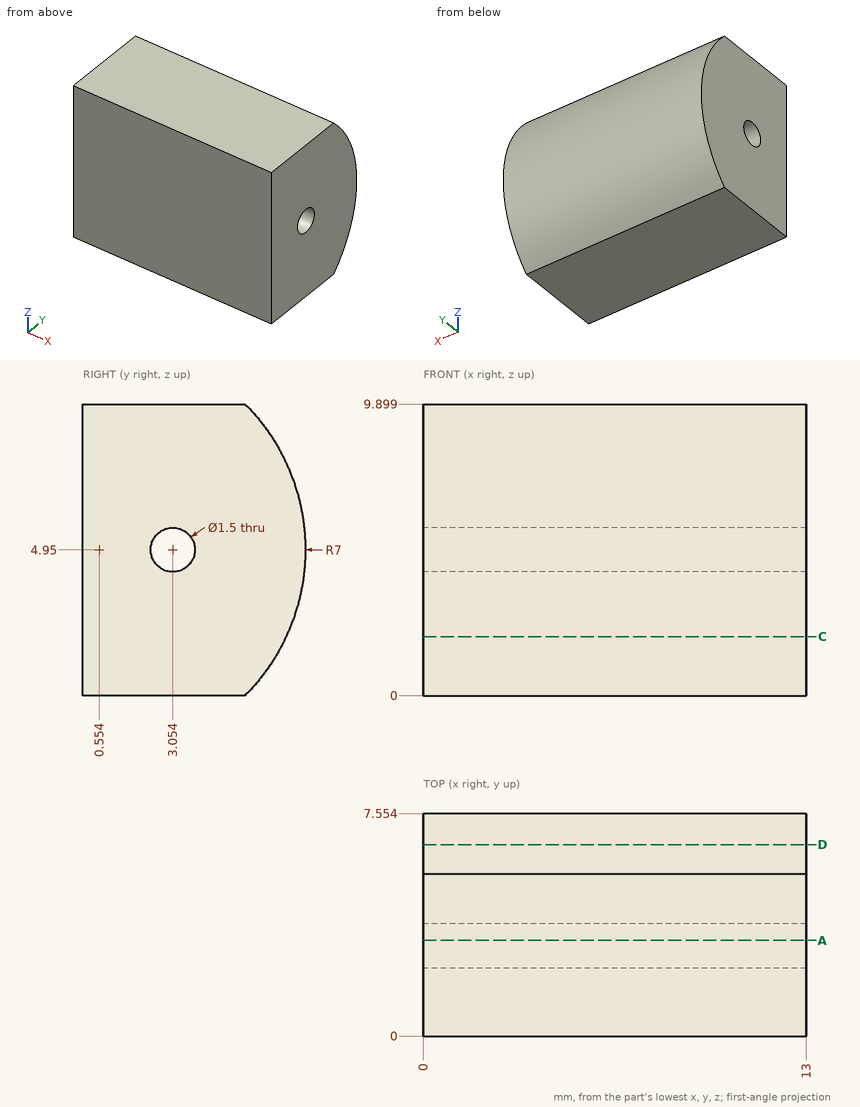
Part print with two shaded views. Sizes in mm from the minimum x, y, z corner. Round coordinates to 2 decimals unless told otherwise and drop trailing zeros. Order: outer loops, then holes, each group sorted by start corner. A loop starts at its lowest first (then second) coordinate and runs counter-clockwise, first axis right, second up. Notation, with made-up numbers: (12.25, -9.75) - (48.25, -9.75) arc R31 cw to (48.25, 29.25) - close; hole circle Ø8 at (-27.75, 37.25). An arc over 180 degrees is marked (long way). Answer as CSV lines item,"result". Start each with the question number.
1. Saw through at A-A, the plane y = 3.25. Write the cut outline in (x, z) (1 decimal).
2. Drill centre lines: L1, parallel to Z at x = 8.5, y = 3; L2, parallel to Y at x = 10, z = 5 (1 decimal); L3, parallel to Y at x = 3.75, z = 4.5 (1 decimal). Where is each one in solid material? Low to high. Write a range as [from, to].
3. Saw through at D-D, the plane y = 6.5. Write the cut outline in (x, z) (1 decimal).
4. Saw through at C-C, the plane z = 2. Write the cut outline in (x, y).
Model answer:
1,outline,"(0, 0) - (13, 0) - (13, 4.2) - (0, 4.2) - close; (0, 5.7) - (13, 5.7) - (13, 9.9) - (0, 9.9) - close"
2,L1,"z = [0, 4.2], [5.7, 9.9]"
2,L2,"y = [0, 2.3], [3.8, 7.6]"
2,L3,"y = [0, 2.5], [3.7, 7.5]"
3,outline,"(0, 1.3) - (13, 1.3) - (13, 8.6) - (0, 8.6) - close"
4,outline,"(0, 0) - (13, 0) - (13, 6.9) - (0, 6.9) - close"
